Could you check a few things on this model? Use its own coordinates, in mm. Face numbers are marked on the shaded views. Round coordinates to 2 decimals unless told otherwise and drop trailing zeros. Loops run counter-clockwise (first coordinate to the right, second up) from the corner with the lowest first, then second, coordinate; pieces in that order, holes last. Notation, with made-up numbers: (33.25, -36.75) -> (59.25, -36.75) arc R14 ccw to (59.25, -24.75) -> close; hole circle Ø9 at (35, 57). An arc over 180 degrees is marked (long way). Write each question's results on one line, items separated by ' | '. Start each with the question number.
1) Imagine slicing it at B-B, the plane z = -117. List the corners of the cut face in (x, y) for me.
2) For P1, Ø5, axis at y = 8.5, z = -59, coming from the -X side; P2, Ø5, axis at y = 17.5, z = -63.5, coming from the +X side; P3, Ø8, axis at y = 3, z = -84.5, coming from the -X side, each with a flat end and sliding along its axis, tell me the tip position at first contact or that it passes through.
3) Imagine slicing it at A-A, the plane y = 69. List the corners of the cut face in (x, z) for me.
4) Imagine slicing it at C-C, the plane x = -181.5. List the corners of the cut face in (y, z) for me, plus the area to 3 significant figures.
5) If I drill on probe 1 along X at (y, z) = (-16, -62); probe 2 along Y at (x, z) = (-119.5, -119.5); probe 3 along X at (y, z) = (54.5, -104), over which ranges is the centre line in solid material (lowest first)?
6) We'd pull the mould along Y, two halves only. Please class the marked faces 1, 2 and 3: pulls with the +Y half, pulls with the -Y half, needs draft (parallel to the pull), parting line crosses it, or undercut.
from build123d import *

# Parameters (mm, degrees)
Y_KSEKLIK_EKSTR_ZYON1_DEPTH       = 80
Y_KSEKLIK_EKSTR_ZYON6_OUTLINE_W   = 9.307663541
Y_KSEKLIK_EKSTR_ZYON6_OUTLINE_H   = 30
Y_KSEKLIK_EKSTR_ZYON6_DEPTH       = 0.619232544
Y_KSEKLIK_EKSTR_ZYON6_START       = -34
Y_KSEKLIK_EKSTR_ZYON6_2_OUTLINE_W = 36
Y_KSEKLIK_EKSTR_ZYON6_2_OUTLINE_H = 30
Y_KSEKLIK_EKSTR_ZYON6_2_DEPTH     = 34
Y_KSEKLIK_EKSTR_ZYON6_START_2     = -85
Y_KSEKLIK_EKSTR_ZYON6_3_OUTLINE_R = 16
Y_KSEKLIK_EKSTR_ZYON6_3_DEPTH     = 30


with BuildPart() as part:
    # izim3 → Y_kseklik-Ekstr_zyon1 (new body)
    with BuildSketch(Plane(origin=(0, 0, 0), x_dir=(1, 0, 0), z_dir=(0, 1, 0))):
        Polygon((-257.534328512, 0.000206653), (-415, 95.915871832), (-415, 135), (0, 135), (0, 0), align=None)
    extrude(amount=Y_KSEKLIK_EKSTR_ZYON1_DEPTH)

    # Y_kseklik-Ekstr_zyon6: read off the stored shape, not the designer's step
    # Y_kseklik-Ekstr_zyon6 outline → Y_kseklik-Ekstr_zyon6 (add)
    with BuildSketch(Plane.YZ):
        with Locations((4.653831771, -70)):
            Rectangle(Y_KSEKLIK_EKSTR_ZYON6_OUTLINE_W, Y_KSEKLIK_EKSTR_ZYON6_OUTLINE_H)
    extrude(amount=Y_KSEKLIK_EKSTR_ZYON6_DEPTH)

    # Y_kseklik-Ekstr_zyon6 2 outline → Y_kseklik-Ekstr_zyon6 2 (add)
    with BuildSketch(Plane(origin=(0, 0, 0), x_dir=(1, 0, 0), z_dir=(0, 1, 0)).offset(Y_KSEKLIK_EKSTR_ZYON6_START)):
        with Locations((-17.380767456, 70)):
            Rectangle(Y_KSEKLIK_EKSTR_ZYON6_2_OUTLINE_W, Y_KSEKLIK_EKSTR_ZYON6_2_OUTLINE_H)
        with Locations((-217.380767456, 70)):
            Rectangle(Y_KSEKLIK_EKSTR_ZYON6_2_OUTLINE_W, Y_KSEKLIK_EKSTR_ZYON6_2_OUTLINE_H)
    extrude(amount=Y_KSEKLIK_EKSTR_ZYON6_2_DEPTH)

    # Y_kseklik-Ekstr_zyon6 3 outline → Y_kseklik-Ekstr_zyon6 3 (cut)
    with BuildSketch(Plane.XY.offset(Y_KSEKLIK_EKSTR_ZYON6_START_2)):
        with BuildLine():
            Line((0.619232544, -34), (0.619232544, -16))
            ThreePointArc((0.619232544, -16), (-4.652845395, -28.727922061), (-17.380767456, -34))
            Line((-17.380767456, -34), (0.619232544, -34))
        make_face()
        with BuildLine():
            Line((-35.380767456, -34), (-17.380767456, -34))
            ThreePointArc((-17.380767456, -34), (-30.108689517, -28.727922061), (-35.380767456, -16))
            Line((-35.380767456, -16), (-35.380767456, -34))
        make_face()
        with Locations((-17.380767456, -16)):
            Circle(Y_KSEKLIK_EKSTR_ZYON6_3_OUTLINE_R)
        with BuildLine():
            Line((-199.380767456, -34), (-199.380767456, -16))
            ThreePointArc((-199.380767456, -16), (-204.652845395, -28.727922061), (-217.380767456, -34))
            Line((-217.380767456, -34), (-199.380767456, -34))
        make_face()
        with BuildLine():
            Line((-235.380767456, -34), (-217.380767456, -34))
            ThreePointArc((-217.380767456, -34), (-230.108689517, -28.727922061), (-235.380767456, -16))
            Line((-235.380767456, -16), (-235.380767456, -34))
        make_face()
        with Locations((-217.380767456, -16)):
            Circle(Y_KSEKLIK_EKSTR_ZYON6_3_OUTLINE_R)
    extrude(amount=Y_KSEKLIK_EKSTR_ZYON6_3_DEPTH, mode=Mode.SUBTRACT)


solid = part.part
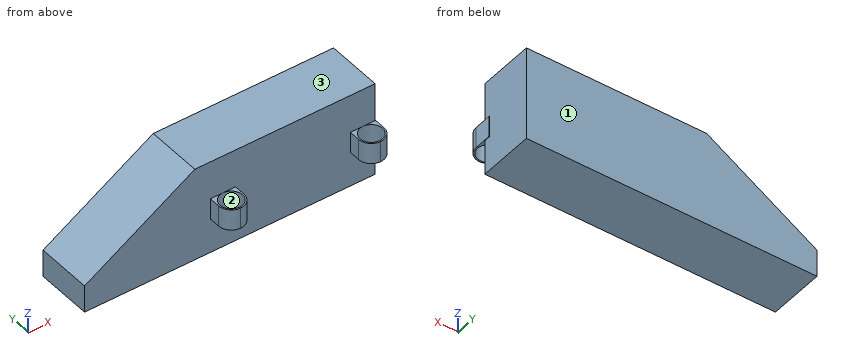
Checked values:
1) outline: (-415, 0) -> (0, 0) -> (0, 80) -> (-415, 80) -> close
2) P1: x = -358.5 | P2: x = 0 | P3: x = -402.83
3) outline: (-415, -135) -> (0, -135) -> (0, 0) -> (-257.53, 0) -> (-415, -95.92) -> close
4) outline: (0, -135) -> (80, -135) -> (80, 0) -> (0, 0) -> close | area: 10,800 mm^2
5) probe 1: -235.38 to -233.38, -201.38 to -199.38, -35.38 to -33.38, -1.38 to 0.62 | probe 2: 0 to 80 | probe 3: -415 to 0
6) face 1: pulls with the +Y half | face 2: undercut | face 3: needs draft
